```python
from build123d import *

# Parameters (mm, degrees)
SKETCH1_W           = 64.5
SKETCH1_H           = 35
BOSS_EXTRUDE1_DEPTH = 75
FILLET1_R           = 2
SKETCH2_R           = 1
FIX_2_DEPTH         = 76
CUT_EXTRUDE2_DEPTH  = 75
CUT_EXTRUDE3_DEPTH  = 75
SKETCH5_W           = 26.25
SKETCH5_H           = 1.5
CUT_EXTRUDE4_DEPTH  = 75
FILLET2_R           = 0.3
SKETCH6_W           = 52.5
SKETCH6_H           = 1.5
BAS_DEPTH           = 76


with BuildPart() as part:
    # Sketch1 → Boss-Extrude1 (new body)
    with BuildSketch(Plane.XY):
        Rectangle(SKETCH1_W, SKETCH1_H)
    extrude(amount=BOSS_EXTRUDE1_DEPTH)

    # Fillet1
    fillet1_edges = [part.edges().sort_by_distance(p)[0] for p in [
        (32.25, -17.5, 37.5),
        (-32.25, -17.5, 37.5),
        (-32.25, 17.5, 37.5),
        (32.25, 17.5, 37.5),
    ]]
    fillet(fillet1_edges, radius=FILLET1_R)

    # Sketch2 → fix 2 (cut, through all)
    with BuildSketch(Plane.XY.offset(75)):
        with Locations((-28.25, 13.5)):
            Circle(SKETCH2_R)
        with Locations((-28.25, -13.5)):
            Circle(SKETCH2_R)
        with Locations((28.25, -13.5)):
            Circle(SKETCH2_R)
        with Locations((28.25, 13.5)):
            Circle(SKETCH2_R)
    extrude(amount=-FIX_2_DEPTH, mode=Mode.SUBTRACT)

    # Sketch3 → Cut-Extrude2 (cut)
    with BuildSketch(Plane.XY.offset(75)):
        Polygon((-27.75, 10.92), (-27.75, 13), (-26.25, 13), (-26.25, 14.5), (0, 14.5), (26.25, 14.5), (26.25, 13), (27.75, 13), (27.75, 10.92), (29.25, 10.92), (29.25, -6.5), (27.75, -6.5), (27.75, -13), (26.25, -13), (26.25, -14.5), (0, -14.5), (-26.25, -14.5), (-26.25, -13), (-27.75, -13), (-27.75, -6.5), (-29.25, -6.5), (-29.25, 10.92), align=None)
    extrude(amount=-CUT_EXTRUDE2_DEPTH, mode=Mode.SUBTRACT)

    # Sketch4 → Cut-Extrude3 (cut)
    with BuildSketch(Plane.XY.offset(75)):
        Polygon((-30, -8), (-28.2, -8), (-28.2, -4.99063684), (28.2, -5.371209777), (28.2, -8), (30, -8), (30, -10.1), (-30, -10.1), align=None)
    extrude(amount=-CUT_EXTRUDE3_DEPTH, mode=Mode.SUBTRACT)

    # Sketch5 → Cut-Extrude4 (cut)
    with BuildSketch(Plane.XY.offset(75)):
        with Locations((13.125, 15.25)):
            Rectangle(SKETCH5_W, SKETCH5_H)
    extrude(amount=-CUT_EXTRUDE4_DEPTH, mode=Mode.SUBTRACT)

    # Fillet2
    fillet2_edges = [part.edges().sort_by_distance(p)[0] for p in [
        (27.75, 12.633974596, 37.5),
        (27.383974596, 13, 37.5),
        (27.383974596, -13, 37.5),
        (27.75, -12.633974596, 37.5),
        (-27.75, -12.633974596, 37.5),
        (-27.383974596, -13, 37.5),
        (-27.383974596, 13, 37.5),
        (-27.75, 12.633974596, 37.5),
    ]]
    fillet(fillet2_edges, radius=FILLET2_R)

    # Sketch6 → bas (cut, through all)
    with BuildSketch(Plane.XY.offset(75)):
        with Locations((0, -15.25)):
            Rectangle(SKETCH6_W, SKETCH6_H)
    extrude(amount=-BAS_DEPTH, mode=Mode.SUBTRACT)


solid = part.part
```
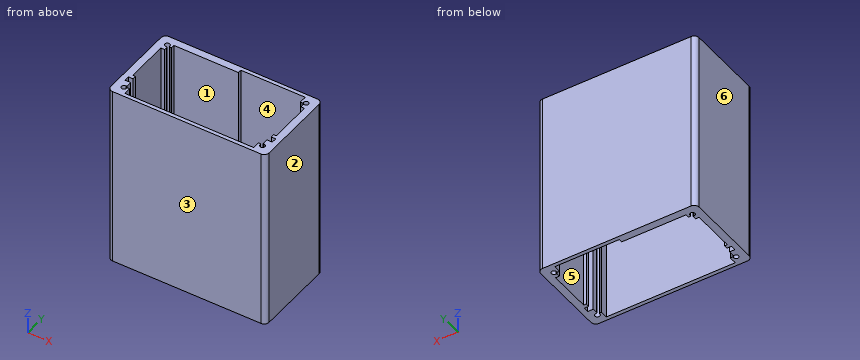
Design review of the part built by this model. Coordinates are the model's own, in mm. Face numbers are marked on the shaded views. A direction names the side the tool comes from. Round coordinates to 2 decimals unless told otherwise and drop trailing zeros. Order: outer loops, then holes, each group sorted by start corner. A loop starts at its lowest first (then second) coordinate and runs counter-clockwise, first axis right, second up. Notation, with made-up numbers: (39, -26) - (79, -26) arc R30 ccw to (79, 6) - close; hole circle Ø9 at (10.5, -20.5). An arc over 180 degrees is marked (long way). Return JSON: item names as keys, results as strings.
Q1. Machinability: for the marked faces 1 and 2, which of the approach directions +Z, -Z, +X, -X, +Y, -Y give a long, thin tool a straight path to every point of the face, cutting with its end or side? Answer none if there is none.
Computed values:
{"face 1": "+Z, -Z", "face 2": "+Z, -Z, +X, +Y, -Y"}
Q2. The part is to be moulded in two halves that separate along Y. For the marked faces 3, 4, 5 and 6, say which applies: pulls with the +Y half, pulls with the -Y half, needs draft (parallel to the pull), parting line crosses it, or undercut.
Computed values:
{"face 3": "pulls with the -Y half", "face 4": "undercut", "face 5": "undercut", "face 6": "needs draft"}
Q3. Consider section A-A on y = -2. Write out the cut boundary in (x, z), plus the area to 3 significant figures.
Computed values:
{"outline": "(-32.25, 0) - (-29.25, 0) - (-29.25, 75) - (-32.25, 75) - close; (29.25, 0) - (32.25, 0) - (32.25, 75) - (29.25, 75) - close", "area": "450 mm2"}
Q4. Wall thickness on L1, parallel to Y at x = 28.25, z = 22; L2, parallel to X at y = -13.5, z = 25.5; L3, parallel to X at y = -8.5, z = 15: over which ranges is each line inside the solid? List them lowest first. Write a range as [from, to].
Computed values:
{"L1": "y = [-17.5, -14.5], [-12.5, -10.1], [-8, -6.5], [10.92, 12.5], [14.5, 17.5]", "L2": "x = [-32.25, -29.25], [-27.25, -26.25], [26.25, 27.25], [29.25, 32.25]", "L3": "x = [-32.25, -30], [30, 32.25]"}
Q5. Consider section B-B on x = -11. Write out the cut boundary in (y, z).
Computed values:
{"outline": "(-17.5, 0) - (-16, 0) - (-16, 75) - (-17.5, 75) - close; (14.5, 0) - (17.5, 0) - (17.5, 75) - (14.5, 75) - close"}
